Geometry: final body of the model. Coordinates: model frame, mm. Face numbers are marked on the shaded views. A direction names the side the tool comes from. Round coordinates to 2 decimals unless told otherwise and drop trailing zeros. Order: outer loops, then holes, each group sorted by start corner. A loop starts at its lowest first (then second) coordinate and runs counter-clockwise, first axis right, second up. Notation, with made-up numbers: M 2,2 L 41,2 A18 ccw 41,6 Z; hole C 41.5,85.25 d5. An arc over 180 degrees is marked long. Put each result on its own line as item: value. Start each with the question number.
1) Access query for the marked faces 4 and 5. Directions: +Z, -Z, +X, -X, +Y, -Y. A direction counts if a zero-diameter tool reaches every point of the face in a straight line with its end or side. Return the directions, or none.
2) Section D-D, the plane y = -32.5. Return loops of the section in (x, z).
3) First-contact query: P1, Ø3, axis at y = -44.5, z = 18.5, coming from the -X side; P2, Ø2.5, axis at x = -75, z = 12.5, coming from the -Y side; P3, Ø4, axis at x = -124, y = -52.5, coming from the -Z side; P4, Ø10, axis at y = -55, z = 11, coming from the -X side. Flat tips, straight axial feed; report the tip coordinate or a pass-through.
4) Section C-C, the plane y = -18. Return loops of the section in (x, z).
5) Draft query along X for the marked faces 1, 2 and 3. Return one class per face: pulls with the +X half, pulls with the -X half, needs draft (parallel to the pull), parting line crosses it, or undercut.
6) Section B-B, the plane x = -101. Return loops of the section in (y, z).
7) Material intervals for probe 1 along Z at (x, y) = (-75, -71); probe 2 along X at (y, z) = (-29, 7.25); probe 3 along Y at (x, z) = (-92, 20.5), sorted ascending. Write a range as [from, to].
8) Section A-A, the plane z = 6.5. Return loops of the section in (x, y), then the cut area to 3 significant figures.
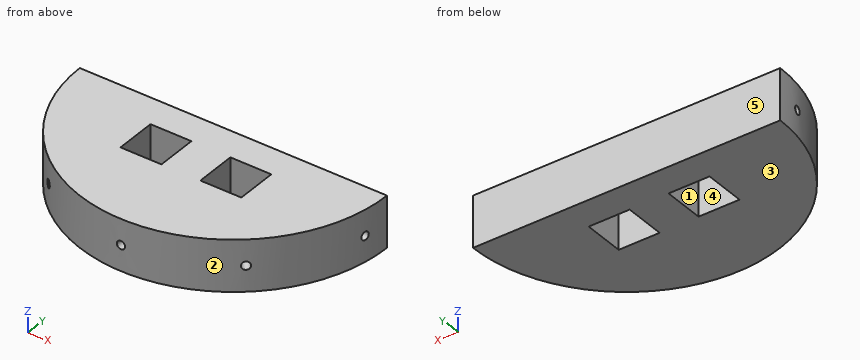
from build123d import *

# Parameters (mm, degrees)
SKETCH1_W           = 20
SKETCH1_H           = 20
BOSS_EXTRUDE1_DEPTH = 25
CIRPATTERN1_COUNT   = 5
CIRPATTERN1_ANGLE   = 160


with BuildPart() as part:
    # Sketch1 → Boss-Extrude1 (new body)
    with BuildSketch(Plane.XY):
        with BuildLine():
            Line((-150, 0), (0, 0))
            ThreePointArc((0, 0), (-75, -75), (-150, 0))
        make_face()
        with Locations((-55.5, -25)):
            Rectangle(SKETCH1_W, SKETCH1_H, mode=Mode.SUBTRACT)
        with Locations((-94.5, -25)):
            Rectangle(SKETCH1_W, SKETCH1_H, mode=Mode.SUBTRACT)
    extrude(amount=BOSS_EXTRUDE1_DEPTH)

    # Sketch4 → Ø4.0mm Dowel Hole2 (revolve, cut)
    with BuildSketch(Plane(origin=(-1.139418524, -13.023613325, 12.5), x_dir=(0.17364817766693047, 0.9848077530122081, 0), z_dir=(0, 0, 1))):
        Polygon((0, 0), (0, 17.201721238), (2, 16), (2, 0.025), (2.025, 0), align=None)
    f_4_0mm_dowel_hole2 = revolve(axis=Axis((5.114110708, -14.126279253, 12.5), (-0.9848077530122081, 0.17364817766693044, 0)), mode=Mode.SUBTRACT)

    # CirPattern1: Ø4.0mm Dowel Hole2 ×5 about axis
    cirpattern1_axis = Axis((-75, 0, 0), (0, 0, -1))
    for i in range(1, CIRPATTERN1_COUNT):
        add(f_4_0mm_dowel_hole2.rotate(cirpattern1_axis, i * CIRPATTERN1_ANGLE / (CIRPATTERN1_COUNT - 1)), mode=Mode.SUBTRACT)


solid = part.part
Result sheet:
1. face 4: +Z, -Z
1. face 5: +Z, -Z, +X, -X, +Y
2. outline: M -142.59,0 L -104.5,0 L -104.5,25 L -142.59,25 Z; M -84.5,0 L -65.5,0 L -65.5,25 L -84.5,25 Z; M -45.5,0 L -7.41,0 L -7.41,25 L -45.5,25 Z
3. P1: stops at x = -136.45
3. P2: stops at y = -58.55
3. P3: stops at z = 0
3. P4: stops at x = -130.9
4. outline: M -147.81,0 L -104.5,0 L -104.5,25 L -147.81,25 Z; M -84.5,0 L -65.5,0 L -65.5,25 L -84.5,25 Z; M -45.5,0 L -2.19,0 L -2.19,25 L -45.5,25 Z
5. face 1: undercut
5. face 2: parting line crosses it
5. face 3: needs draft
6. outline: M -70.35,0 L -35,0 L -35,25 L -70.35,25 Z; M -15,0 L 0,0 L 0,25 L -15,25 Z
7. probe 1: z = [0, 10.5], [14.5, 25]
7. probe 2: x = [-144.17, -104.5], [-84.5, -65.5], [-45.5, -5.83]
7. probe 3: y = [-73.05, -35], [-15, 0]
8. outline: M -150,0 A75 ccw 0,0 Z; hole M -104.5,-35 L -84.5,-35 L -84.5,-15 L -104.5,-15 Z; hole M -65.5,-35 L -45.5,-35 L -45.5,-15 L -65.5,-15 Z
8. area: 8,040 mm2
